Geometry check sheet. Reference: drawing and pictorial views, mm from the part's lowest x, y, z. A direction names the side the tool comes from. Round coordinates to 2 decimals unless told otherwise and drop trailing zeros. Order: outer loops, then holes, each group sorted by start corner. A loop starts at its lowest first (then second) coordinate and runs counter-clockwise, first axis right, second up.
(1) Set-up check for the marked faces 1 and 2: record each of +Z, -Z, +X, -X, +Y, -Y from which the full face is reachable in a straight line by a thin tool's end or side.
(2) Cross-section at C-C on x = 15.5. Enter the section's corners in (y, z).
(3) Cross-section at D-D on y = 18.5. Enter the section's corners in (x, z).
(4) Cross-section at B-B on y = 34. Enter the section's corners in (x, z).
(5) Cross-section at A-A on x = 3. Enter the section's corners in (y, z).
(6) Thickness scan on L1, parallel to X at y = 3.25, z = 6; L2, parallel to Y at x = 4.75, z = 11; L3, parallel to Z at x = 8, y = 4. Record the ranges inside material, lowest first.
(7) Gauge pin test, flat ends, axial feed: P1, Ø4.5, axis at x = 8, z = 24, coming from the -Y side; P2, Ø2, axis at x = 23, z = 24, coming from the +Y side; P3, Ø2.5, axis at x = 23, z = 6, coming from the -Y side; P4, Ø2.5, axis at x = 23, z = 24, coming from the +Y side. Record the tip position at first contact, or that the pin passes through.
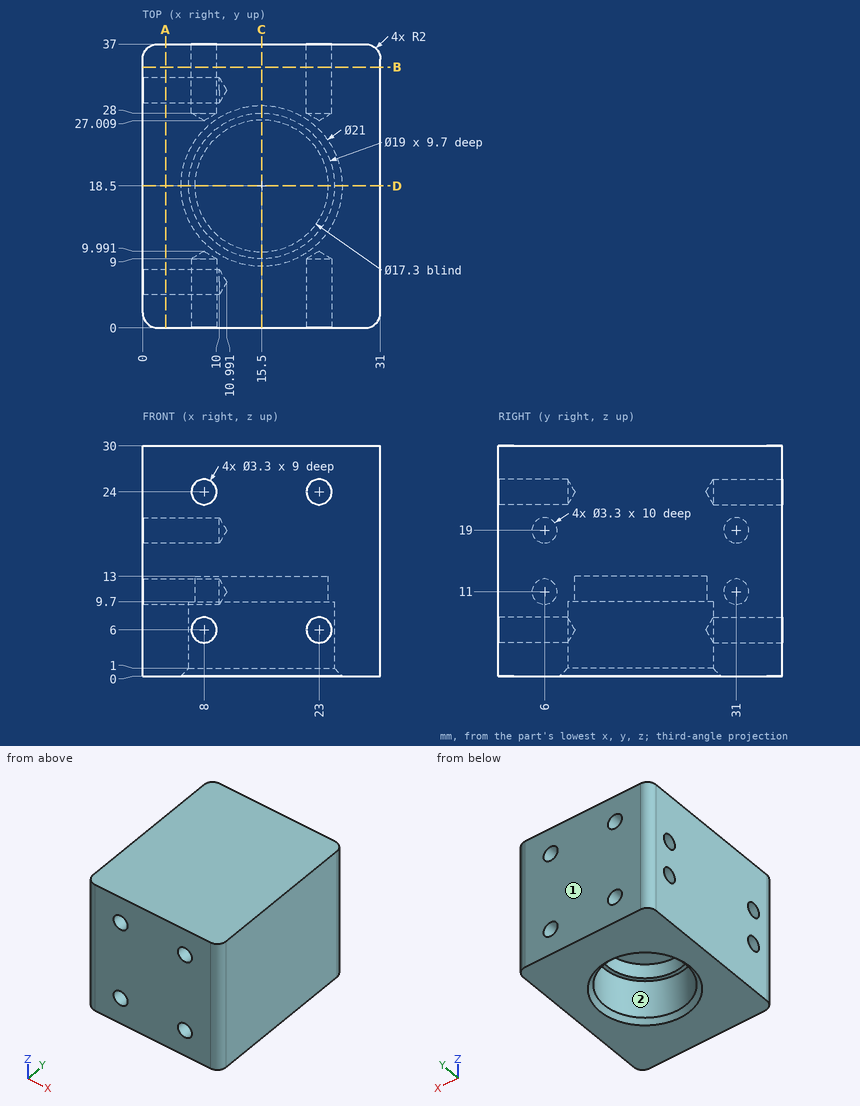
Found:
1. face 1: +Z, -Z, +X, -X, +Y
1. face 2: -Z
2. outline: (0, 0) - (8, 0) - (9, 1) - (9, 9.7) - (9.85, 9.7) - (9.85, 13) - (27.15, 13) - (27.15, 9.7) - (28, 9.7) - (28, 1) - (29, 0) - (37, 0) - (37, 30) - (0, 30) - close
3. outline: (0, 0) - (5, 0) - (6, 1) - (6, 9.7) - (6.85, 9.7) - (6.85, 13) - (24.15, 13) - (24.15, 9.7) - (25, 9.7) - (25, 1) - (26, 0) - (31, 0) - (31, 30) - (0, 30) - close
4. outline: (0, 0) - (31, 0) - (31, 30) - (0, 30) - close; hole circle Ø3.3 at (8, 6); hole circle Ø3.3 at (8, 24); hole circle Ø3.3 at (23, 6); hole circle Ø3.3 at (23, 24)
5. outline: (0, 0) - (37, 0) - (37, 30) - (0, 30) - close; hole circle Ø3.3 at (6, 11); hole circle Ø3.3 at (6, 19); hole circle Ø3.3 at (31, 11); hole circle Ø3.3 at (31, 19)
6. L1: x = 0 to 6.35, 9.65 to 21.35, 24.65 to 31
6. L2: y = 0 to 4.35, 7.65 to 29.35, 32.65 to 37
6. L3: z = 0 to 4.35, 7.65 to 22.35, 25.65 to 30
7. P1: stops at y = 0
7. P2: stops at y = 27.61
7. P3: stops at y = 9.24
7. P4: stops at y = 27.76
